```python
from build123d import *

# Parameters (mm, degrees)
SKETCH1_W           = 59.6
SKETCH1_H           = 30
SKETCH1_R           = 2.35
SKETCH1_W_2         = 40.5
SKETCH1_H_2         = 21
BOSS_EXTRUDE1_DEPTH = 10
FILLET1_R           = 2


with BuildPart() as part:
    # Sketch1 → Boss-Extrude1 (new body)
    with BuildSketch(Plane.XY):
        Rectangle(SKETCH1_W, SKETCH1_H)
        with Locations((-24.8, 5)):
            Circle(SKETCH1_R, mode=Mode.SUBTRACT)
        with Locations((24.8, 5)):
            Circle(SKETCH1_R, mode=Mode.SUBTRACT)
        with Locations(Location((24.8, -5, 0), (0, 0, 180))):
            Circle(SKETCH1_R, mode=Mode.SUBTRACT)
        with Locations(Location((-24.8, -5, 0), (0, 0, 180))):
            Circle(SKETCH1_R, mode=Mode.SUBTRACT)
        Rectangle(SKETCH1_W_2, SKETCH1_H_2, mode=Mode.SUBTRACT)
    extrude(amount=BOSS_EXTRUDE1_DEPTH)

    # Fillet1
    fillet1_edges = [part.edges().sort_by_distance(p)[0] for p in [
        (0, 15, 10),
        (0, 15, 0),
        (0, -15, 0),
        (-29.8, 15, 5),
        (29.8, 15, 5),
        (29.8, -15, 5),
        (-29.8, -15, 5),
        (0, -15, 10),
    ]]
    fillet(fillet1_edges, radius=FILLET1_R)


solid = part.part
```
Input: part model. Units: mm. Frame: model coordinates. A direction names the side the tool comes from. Round coordinates to 2 decimals unless told otherwise and drop trailing zeros. Loops run counter-clockwise (first coordinate to the right, second up) from the corner with the lowest first, then second, coordinate; pieces in that order, holes last. Notation, with made-up numbers: M -23.5,14.25 L 31.5,14.25 A13 cw 31.5,31.25 Z; hole C 18,30.5 d6. An arc over 180 degrees is marked long. Answer in a Markdown table with one row per item. Add a question column.
1. Section D-D (y = 5). Output: boundary loops of the cut face in (x, z), and give its area (3 significant figures).
2. Ray query, probe 1 along X at (y, z) = (-4.75, 6.75); probe 2 along Y at (x, z) = (-24.8, 2); probe 3 along Y at (x, z) = (1.5, 2.75). Return the intervals inside material, ascending.
3. Section A-A (y = -1.75). Output: boundary loops of the cut face in (x, z).
4. Section B-B (x = -12). Output: boundary loops of the cut face in (y, z), and give its area (3 significant figures).
5. Section C-C (z = 3.25). Output: boundary loops of the cut face in (x, y).
6. Contact query for a flat-ended pin moving along its axis: pin 1 (4 mm diameter, centred on x = 24.8, y = -5, fed in from +Z). Output: stop coordinate, or through.
7. Mould query, pull axis Y, two halves, no side actions, for faces 3 (the face through (-29.23, 14.4, 5.07)), 4 (the face through (22.63, -4.1, 4.93)), 5 (the face through (0.42, -14.43, 9.4)), 6 (the face through (-7, -11, 10)). Classes: released by +Y, released by -Y, zero draft, split by the parting line, or undercut.
8. Set-up query: faces 1 (the face through (-7, -11, 0)), 2 (the face through (-20.25, 0, 5)). Return all of +Z, -Z, +X, -X, +Y, -Y with unobstructed straight access to the full face (end or side cutting, diameter ignored); none if empty.
Values follow:
| question | item | result |
|---|---|---|
| 1 | outline | M -29.8,0 L -27.15,0 L -27.15,10 L -29.8,10 Z; M -22.45,0 L -20.25,0 L -20.25,10 L -22.45,10 Z; M 20.25,0 L 22.45,0 L 22.45,10 L 20.25,10 Z; M 27.15,0 L 29.8,0 L 29.8,10 L 27.15,10 Z |
| 1 | area | 97.0 mm^2 |
| 2 | probe 1 | -29.8 to -27.14, -22.46 to -20.25, 20.25 to 22.46, 27.14 to 29.8 |
| 2 | probe 2 | -15 to -7.35, -2.65 to 2.65, 7.35 to 15 |
| 2 | probe 3 | -15 to -10.5, 10.5 to 15 |
| 3 | outline | M -29.8,0 L -20.25,0 L -20.25,10 L -29.8,10 Z; M 20.25,0 L 29.8,0 L 29.8,10 L 20.25,10 Z |
| 4 | outline | M -15,2 A2 ccw -13,0 L -10.5,0 L -10.5,10 L -13,10 A2 ccw -15,8 Z; M 10.5,0 L 13,0 A2 ccw 15,2 L 15,8 A2 ccw 13,10 L 10.5,10 Z |
| 4 | area | 86.6 mm^2 |
| 5 | outline | M -29.8,-13 A2 ccw -27.8,-15 L 27.8,-15 A2 ccw 29.8,-13 L 29.8,13 A2 ccw 27.8,15 L -27.8,15 A2 ccw -29.8,13 Z; hole C -24.8,-5 d4.7; hole C -24.8,5 d4.7; hole M -20.25,-10.5 L 20.25,-10.5 L 20.25,10.5 L -20.25,10.5 Z; hole C 24.8,-5 d4.7; hole C 24.8,5 d4.7 |
| 6 | pin 1 | through |
| 7 | face 3 | released by +Y |
| 7 | face 4 | undercut |
| 7 | face 5 | released by -Y |
| 7 | face 6 | zero draft |
| 8 | face 1 | -Z, +X, -X, +Y, -Y |
| 8 | face 2 | +Z, -Z |
